```python
from build123d import *

# Parameters (mm, degrees)
F1_DEPTH = 60
F2_R     = 29.99999
F3_R     = 15
F4_DEPTH = 78.3
F5_R     = 5
F6_DEPTH = 25


# Not quite as in the source:
# - a fillet or chamfer is up to 0.001 mm smaller than in the source, because OpenCascade refuses the exact size


with BuildPart() as f1:
    # F0 (on Front) → F1 (new body)
    with BuildSketch(Plane.XZ):
        Polygon((80, 0), (0, 0), (0, -10), (77.3205080757, -10), (126.9615242271, -38.6602540378), (131.9615242271, -30), align=None)
    extrude(amount=-F1_DEPTH)

    # F2 (radius 30 in the source; OpenCascade refuses exactly that, so slightly less here)
    f2_edges = [f1.edges().sort_by_distance(p)[0] for p in [
        (129.461524, 60, -34.330127),
        (129.461524, 0, -34.330127),
    ]]
    fillet(f2_edges, radius=F2_R)

    # F3 (on face) → F4 (cut)
    with BuildSketch(Plane(origin=(20, 0, 34.6410161514), x_dir=(0.8660254038, 0, -0.5), z_dir=(0.5, 0, 0.8660254038))):
        with Locations((98.4833240509, 30.9668332338)):
            Circle(F3_R)
    extrude(amount=-F4_DEPTH, mode=Mode.SUBTRACT)

    # F5 (on face) → F6 (cut)
    with BuildSketch(Plane.XY):
        with Locations((12, 47)):
            Circle(F5_R)
        with Locations((12, 12)):
            Circle(F5_R)
        with Locations((67, 12)):
            Circle(F5_R)
        with Locations((67, 47)):
            Circle(F5_R)
    extrude(amount=-F6_DEPTH, mode=Mode.SUBTRACT)


solid = f1.part
```
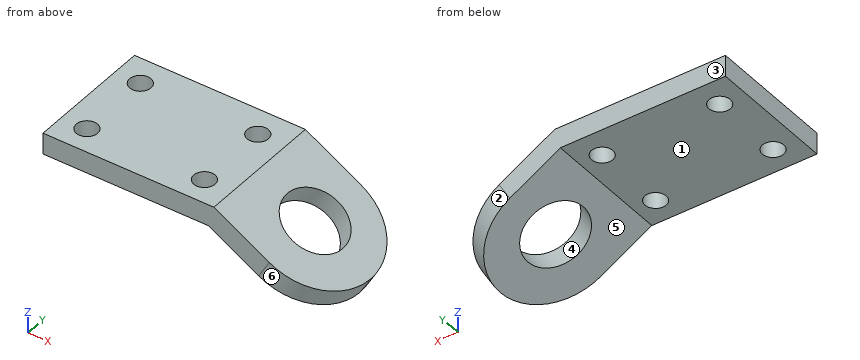
Read the model definition and answer for the solid it produces. Units are mm, in the model's axes. Face numbers are marked on the shaded views. A direction names the side the tool comes from. Coordinates: 2 decimals unless noted, no trailing zeros. Write each loop counter-clockwise with the first axis right and the second up, starting at its lowest first coordinate (ties: lowest second). Pieces come first, ordered by that corner, then holes. Notation, with made-up numbers: (-33, 47.5) -> (-6, 47.5) arc R21 cw to (-6, 70.5) -> close; hole circle Ø7 at (-12, 12). An arc over 180 degrees is marked (long way). Return JSON: item names as keys, results as strings.
1. Find the intervals of material crossed by line 1 along Y through (x, z) = (67.5, -4); line 2 along Z through (x, y) = (26.5, 40.5); line 3 along X through (y, z) = (30.5, -29), in increasing order. Write a range as from..to.
Found:
{"line 1": "0..7.03, 16.97..42.03, 51.97..60", "line 2": "-10..0", "line 3": "114.29..130.23"}
2. Each of these flat-tipped pins is pushed along its axis until it touches: P1, Ø1, axis at y = 26, z = -5, coming from the +X side; P2, Ø6, axis at x = 67, y = 12, coming from the +Z side; P3, Ø1, axis at x = 91, y = 53, coming from the -Z side; P4, Ø16, axis at x = 12, y = 47, coming from the -Z side. Where does it stop, or does it pass through?
Found:
{"P1": "x = 89.53", "P2": "through", "P3": "z = -18.19", "P4": "z = -10"}
3. A cutting plane is placed at B-B (y = 33.5). Determine the outline of the cut face in (x, z), and give its area (3 significant figures).
Found:
{"outline": "(0, -10) -> (77.32, -10) -> (87.49, -15.87) -> (92.49, -7.21) -> (80, 0) -> (0, 0) -> close; (113.09, -30.65) -> (126.78, -38.56) -> (131.78, -29.9) -> (118.09, -21.99) -> close", "area": "1,080 mm2"}
4. A tool of negligible diameter and unlimited length cuts with its end or side. For the marked faces 1 and 2, from which of +Z, -Z, +X, -X, +Y, -Y can it reach the whole face along a straight path? Write none if from no direction.
Found:
{"face 1": "-Z, -X, +Y, -Y", "face 2": "-Z, +X, +Y"}
5. A cutting plane is placed at A-A (x = 67). Determine the outline of the cut face in (y, z).
Found:
{"outline": "(0, -10) -> (7, -10) -> (7, 0) -> (0, 0) -> close; (17, -10) -> (42, -10) -> (42, 0) -> (17, 0) -> close; (52, -10) -> (60, -10) -> (60, 0) -> (52, 0) -> close"}
6. A cutting plane is placed at C-C (y = 12). Determine the outline of the cut face in (x, z).
Found:
{"outline": "(0, -10) -> (7, -10) -> (7, 0) -> (0, 0) -> close; (17, -10) -> (62, -10) -> (62, 0) -> (17, 0) -> close; (72, -10) -> (77.32, -10) -> (121.77, -35.66) -> (126.77, -27) -> (80, 0) -> (72, 0) -> close"}
7. A cutting plane is placed at D-D (z = -3.5). Determine the outline of the cut face in (x, y), and give its area (3 significant figures).
Found:
{"outline": "(0, 0) -> (86.06, 0) -> (86.06, 60) -> (0, 60) -> close; hole circle Ø10 at (12, 12); hole circle Ø10 at (12, 47); hole circle Ø10 at (67, 12); hole circle Ø10 at (67, 47)", "area": "4,850 mm2"}
8. Determine the mould class of the marked faces 3, 4, 5 and 6 for opening direction Y: pulls with the +Y half, pulls with the -Y half, needs draft (parallel to the pull), parting line crosses it, or undercut.
Found:
{"face 3": "pulls with the +Y half", "face 4": "undercut", "face 5": "needs draft", "face 6": "pulls with the -Y half"}
